from build123d import *

# Parameters (mm, degrees)
BOSS_EXTRUDE1_DEPTH = 327
SKETCH2_R           = 1.95
CUT_EXTRUDE1_DEPTH  = 2
SKETCH3_R           = 1.95
CUT_EXTRUDE2_DEPTH  = 2
SKETCH5_W           = 16.3
SKETCH5_H           = 1.3
CUT_EXTRUDE4_DEPTH  = 20
SKETCH6_W           = 16.3
SKETCH6_H           = 16.3
BOSS_EXTRUDE3_DEPTH = 1.3
SKETCH7_W           = 16.3
SKETCH7_H           = 16.3
BOSS_EXTRUDE4_DEPTH = 1.3
SKETCH8_R           = 1.95
CUT_EXTRUDE7_DEPTH  = 350


with BuildPart() as part:
    # Sketch1 → Boss-Extrude1 (new body)
    with BuildSketch(Plane(origin=(0, 0, 0), x_dir=(1, 0, 0), z_dir=(0, 1, 0))):
        Polygon((0, 0), (0, 16.3), (1, 16.3), (1, 1), (16.3, 1), (16.3, 0), align=None)
    extrude(amount=BOSS_EXTRUDE1_DEPTH)

    # Sketch2 → Cut-Extrude1 (cut)
    with BuildSketch(Plane.XY):
        with Locations((12.4, 197)):
            Circle(SKETCH2_R)
        with Locations((12.4, 191)):
            Circle(SKETCH2_R)
        with Locations((12.4, 136)):
            Circle(SKETCH2_R)
        with Locations((12.4, 130)):
            Circle(SKETCH2_R)
        with Locations((12.4, 75)):
            Circle(SKETCH2_R)
        with Locations((12.4, 69)):
            Circle(SKETCH2_R)
        with Locations((12.4, 14)):
            Circle(SKETCH2_R)
        with Locations((12.4, 8)):
            Circle(SKETCH2_R)
        with Locations((12.4, 319)):
            Circle(SKETCH2_R)
        with Locations((12.4, 313)):
            Circle(SKETCH2_R)
        with Locations((12.4, 258)):
            Circle(SKETCH2_R)
        with Locations((12.4, 252)):
            Circle(SKETCH2_R)
    extrude(amount=-CUT_EXTRUDE1_DEPTH, mode=Mode.SUBTRACT)

    # Sketch3 → Cut-Extrude2 (cut)
    with BuildSketch(Plane.ZY):
        with Locations((-12.4, 313)):
            Circle(SKETCH3_R)
        with Locations((-12.4, 258)):
            Circle(SKETCH3_R)
        with Locations((-12.4, 252)):
            Circle(SKETCH3_R)
        with Locations((-12.4, 197)):
            Circle(SKETCH3_R)
        with Locations((-12.4, 191)):
            Circle(SKETCH3_R)
        with Locations((-12.4, 136)):
            Circle(SKETCH3_R)
        with Locations((-12.4, 130)):
            Circle(SKETCH3_R)
        with Locations((-12.4, 75)):
            Circle(SKETCH3_R)
        with Locations((-12.4, 69)):
            Circle(SKETCH3_R)
        with Locations((-12.4, 8)):
            Circle(SKETCH3_R)
        with Locations((-12.4, 14)):
            Circle(SKETCH3_R)
        with Locations((-12.4, 319)):
            Circle(SKETCH3_R)
    extrude(amount=-CUT_EXTRUDE2_DEPTH, mode=Mode.SUBTRACT)

    # Sketch5 → Cut-Extrude4 (cut)
    with BuildSketch(Plane.ZY):
        with Locations((-8.15, 0.65)):
            Rectangle(SKETCH5_W, SKETCH5_H)
        with Locations((-8.15, 326.35)):
            Rectangle(SKETCH5_W, SKETCH5_H)
    extrude(amount=-CUT_EXTRUDE4_DEPTH, mode=Mode.SUBTRACT)

    # Sketch6 → Boss-Extrude3 (add)
    with BuildSketch(Plane(origin=(0, 325.7, 0), x_dir=(1, 0, 0), z_dir=(0, 1, 0))):
        with Locations((8.15, 8.15)):
            Rectangle(SKETCH6_W, SKETCH6_H)
    extrude(amount=-BOSS_EXTRUDE3_DEPTH)

    # Sketch7 → Boss-Extrude4 (add)
    with BuildSketch(Plane.XZ.offset(-1.3)):
        with Locations((8.15, -8.15)):
            Rectangle(SKETCH7_W, SKETCH7_H)
    extrude(amount=-BOSS_EXTRUDE4_DEPTH)

    # Sketch8 → Cut-Extrude7 (cut)
    with BuildSketch(Plane.XZ.offset(-1.3)):
        with Locations(Location((12.4, -6.3, 0), (0, 0, 270))):
            Circle(SKETCH8_R)
        with Locations(Location((6.3, -12.4, 0), (0, 0, 270))):
            Circle(SKETCH8_R)
    extrude(amount=-CUT_EXTRUDE7_DEPTH, mode=Mode.SUBTRACT)


solid = part.part
Work out the finished part from the listing and answer in its coordinate system (mm). A direction names the side the tool comes from. Round coordinates to 2 decimals unless told otherwise and drop trailing zeros. Loops run counter-clockwise (first coordinate to the right, second up) from the corner with the lowest first, then second, coordinate; pieces in that order, holes last. Notation, with made-up numbers: (11.25, 15) - (28.25, 15) arc R8 cw to (28.25, 27) - close; hole circle Ø6 at (16, 46). An arc over 180 degrees is marked (long way). Use one line per item in the form item = value. Start each with the question number.
(1) Flat-ended cylindrical pins translate along their axes: P1, Ø4, axis at x = 5, y = 199, coming from the -Z side; P2, Ø4.5, axis at y = 197, z = -12.4, coming from the +X side. Find the tip coordinate at first contact, or state that the pin passes through.
(2) Which of the six approach directions +Z, -Z, +X, -X, +Y, -Y give full straight-line access (tool end or side, diameter ignored) to faces 1 (the face through (9, 2.6, -9)), 2 (the face through (0.3, 162.7, -16.3))?
(3) Consider line 1 (Y direction, x = 9.5, z = -2.75); line 2 (Z direction, x = 0.6, y = 197); line 3 (X direction, y = 258, z = -0.65). Determine where each line is inside the solid, lowest interval first.
(4) Find section A-A on y = 294.5. Determine the outline of the cut face in (x, z), and give its area (3 significant figures).
Answer list:
q1.P1 = -1
q1.P2 = 1
q2.face_1 = -Z, +X
q2.face_2 = -Z, +X, -X, +Y, -Y
q3.line_1 = 1.3 to 2.6, 324.4 to 325.7
q3.line_2 = -16.3 to -14.35, -10.45 to 0
q3.line_3 = 0 to 10.45, 14.35 to 16.3
q4.outline = (0, -16.3) - (1, -16.3) - (1, -1) - (16.3, -1) - (16.3, 0) - (0, 0) - close
q4.area = 31.6 mm^2
